Here's the drawing with two shaded views (mm, measured from the low corner). I have some questions. Give positions to 0.01 mm unless a question says otherwise; leave off trailing zeros. Put each result on its own line as item: value. Start each with the question number.
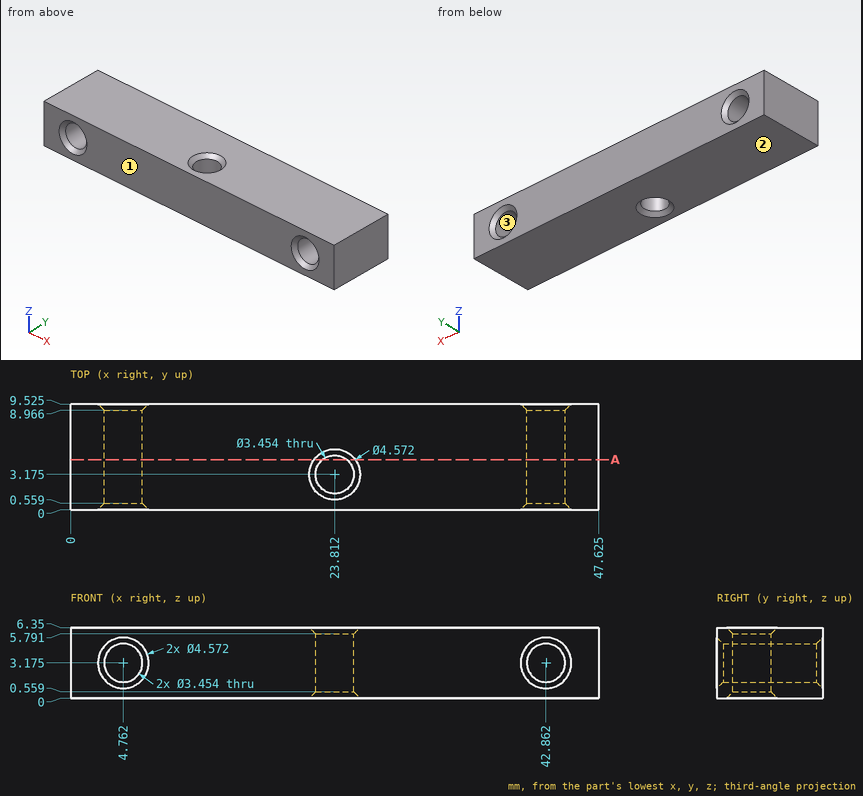
1) Thinking about a two-plate mould opening in Z: for the marked faces 1, 2 and 3, which applies, released by +Z, released by -Z, zero draft, split by the parting line, or undercut?
2) I want a section at A-A, the plane y = 4.5. State how many separate pieces and enclosed holes the cut face has, and give its area (3 significant figures).
3) I need wall thicknesses on probe 1 along Z at (x, y) = (43, 8); probe 2 along X at (y, z) = (5, 3) (1 decimal); probe 3 along X at (y, z) = (8, 2.75) (1 decimal). Which ranges of each line are inside material? Lowest first, please.
Established:
1. face 1: zero draft
1. face 2: released by -Z
1. face 3: undercut
2. separate pieces: 2
2. enclosed holes: 2
2. area: 269 mm2
3. probe 1: z = 0 to 1.45, 4.9 to 6.35
3. probe 2: x = 0 to 3, 6.5 to 41.1, 44.6 to 47.6
3. probe 3: x = 0 to 3.1, 6.4 to 41.2, 44.5 to 47.6
